Here's how the part is built. I have some questions about the finished solid (model axes, mm). A direction names the side the tool comes from. Round coordinates to 2 decimals unless told otherwise and drop trailing zeros. Write each loop counter-clockwise with the first axis right and the second up, starting at its lowest first coordinate (ties: lowest second). Pieces come first, ordered by that corner, then holes. Notation, with made-up numbers: (64.25, -33) -> (114.25, -33) arc R12 cw to (114.25, -15) -> close; hole circle Ø7 at (45, 48.25). An arc over 180 degrees is marked (long way). Answer as CSV lines item,"result".
```python
from build123d import *

# Parameters (mm, degrees)
BOSS_EXTRUDE1_DEPTH      = 50
BOSS_EXTRUDE1_DEPTH_BACK = 50
FILLET1_R                = 50
CUT_EXTRUDE1_DEPTH       = 298.062325719
CUT_EXTRUDE1_DEPTH_BACK  = 298.062325719
HOLE1_D                  = 50


with BuildPart() as part:
    # Sketch1 → Boss-Extrude1 (new, two sides: drawn at the far end of the back side and taken through both)
    with BuildSketch(Plane(origin=(0, 0, 0), x_dir=(1, 0, 0), z_dir=(0, 1, 0)).offset(-BOSS_EXTRUDE1_DEPTH_BACK)):
        with BuildLine():
            Line((-50, -25), (0, -25))
            ThreePointArc((0, -25), (25, 0), (0, 25))
            Line((0, 25), (-50, 25))
            ThreePointArc((-50, 25), (-35.355339059, 60.355339059), (0, 75))
            Line((0, 75), (175.219958145, 75))
            Line((175.219958145, 75), (175.219958145, 15))
            Line((175.219958145, 15), (275.219958145, 15))
            Line((275.219958145, 15), (275.219958145, -15))
            Line((275.219958145, -15), (175.219958145, -15))
            Line((175.219958145, -15), (175.219958145, -75))
            Line((175.219958145, -75), (0, -75))
            ThreePointArc((0, -75), (-35.355339059, -60.355339059), (-50, -25))
        make_face()
    extrude(amount=BOSS_EXTRUDE1_DEPTH + BOSS_EXTRUDE1_DEPTH_BACK)

    # Fillet1
    fillet1_edges = [part.edges().sort_by_distance(p)[0] for p in [
        (275.219958145, 50, 0),
        (275.219958145, -50, 0),
    ]]
    fillet(fillet1_edges, radius=FILLET1_R - 0.0001)  # a hair under: the kernel refuses the full size

    # Sketch4 → Cut-Extrude1 (cut, two sides: drawn at the far end of the back side and taken through both)
    with BuildSketch(Plane(origin=(0, 0, 25), x_dir=(-1, 0, 0), z_dir=(0, 0, -1)).offset(-CUT_EXTRUDE1_DEPTH_BACK)):
        Polygon((0, 20), (50, 20), (50, 50), (0, 50), (-31.919958145, 50), (-31.919958145, 20), align=None)
        Polygon((0, -20), (50, -20), (50, -50), (0, -50), (-31.919958145, -50), (-31.919958145, -20), align=None)
    extrude(amount=CUT_EXTRUDE1_DEPTH + CUT_EXTRUDE1_DEPTH_BACK, mode=Mode.SUBTRACT)

    # Hole1 (through all)
    with Locations(Plane(origin=(0, 0, -15), x_dir=(-1, 0, 0), z_dir=(0, 0, -1))):
        with Locations((-225.219958145, 0)):
            Hole(HOLE1_D / 2)


solid = part.part
```
1. If I drill on line 1 (Y direction, x = -0.5, z = -52); line 2 (Z direction, x = 192.5, y = 0.5); line 3 (X direction, y = -29, z = -62), over which ranges is the centre line in solid material (lowest first)?
Numbers:
line 1,"y = -20 to 20"
line 2,"z = -15 to 15"
line 3,"x = 31.92 to 175.22"
2. Suppose I cut it at C-C on x = 209. Please give me the cut outline in (y, z).
Numbers:
outline,"(-50, -15) -> (-19.02, -15) -> (-19.02, 15) -> (-50, 15) -> close; (19.02, -15) -> (50, -15) -> (50, 15) -> (19.02, 15) -> close"
3. On a 3-axis mill with a long thin cutter (end or side, diameter ignored), from which of +Z, -Z, +X, -X, +Y, -Y can I reach the whole of each face in a straight line? I mean faces 1 (the face through (31.92, 35, 1)), 2 (the face through (215, -23, 15)), 3 (the face through (175.22, -1, -45)), 4 (the face through (31.92, -35, 1)), 5 (the face through (-25, 0, 25)). Say none if no direction works.
Numbers:
face 1,"+Z, -Z, -X, +Y"
face 2,"+Z, +X, +Y, -Y"
face 3,"-Z, +X, +Y, -Y"
face 4,"+Z, -Z, -X, -Y"
face 5,"-X, +Y, -Y"
4. If we mould it in two halves opening along Z, with no side actions, what happens to faces 6 (the face through (18, -20, 18)), 7 (the face through (108, -1, 75)), 8 (the face through (-25, 0, -25))? For each: released by +Z, released by -Z, zero draft, split by the parting line, or undercut.
Numbers:
face 6,"zero draft"
face 7,"released by +Z"
face 8,"undercut"
5. Suppose I cut it at B-B on y = 8. Please give me the cut outline in (x, z).
Numbers:
outline,"(-50, -25) arc R50 ccw to (0, -75) -> (175.22, -75) -> (175.22, -15) -> (201.53, -15) -> (201.53, 15) -> (175.22, 15) -> (175.22, 75) -> (0, 75) arc R50 ccw to (-50, 25) -> (0, 25) arc R25 cw to (0, -25) -> close; (248.91, -15) -> (274.58, -15) -> (274.58, 15) -> (248.91, 15) -> close"
6. Suppose I cut it at D-D on y = -9.5. Please give me the cut outline in (x, z).
Numbers:
outline,"(-50, -25) arc R50 ccw to (0, -75) -> (175.22, -75) -> (175.22, -15) -> (202.1, -15) -> (202.1, 15) -> (175.22, 15) -> (175.22, 75) -> (0, 75) arc R50 ccw to (-50, 25) -> (0, 25) arc R25 cw to (0, -25) -> close; (248.34, -15) -> (274.31, -15) -> (274.31, 15) -> (248.34, 15) -> close"
7. For pin 1 Ø2 at (x, y) = (200, 40) entering from -Z; pin 2 Ø24 at (y, z) = (31, 9.5) entering from -X; pin 3 Ø1 at (y, z) = (17.5, 6) entering from -X, each with a flat end and sliding along its axis, tell me the tip position at first contact or that it passes through.
Numbers:
pin 1,"stops at z = -15"
pin 2,"stops at x = 20.51"
pin 3,"stops at x = 24.14"
